The listing builds one solid part. Answer for the finished solid, in the listing's coordinates (mm). Coordinates: 2 decimals unless noted, no trailing zeros. Loops run counter-clockwise (first coordinate to the right, second up) from the corner with the lowest first, then second, coordinate; pieces in that order, holes last. Notation, with made-up numbers: M 53,60 L 92,60 A19 cw 92,77 Z; hole C 4,-20 d4. An arc over 180 degrees is marked long. Answer as a JSON object with one key per item and string values. Group by question number.
1. A cutting plane is placed at B-B on x = -4.5. State how many separate pieces and enclosed holes the cut face has, and give its area (3 significant figures).
2. Straight lines are drawn through the part: L1, parallel to X at y = 1.25, z = 16.5; L2, parallel to X at y = 1.3, z = 67; L3, parallel to X at y = 1.1, z = 97.5. For each, find the intervals that lie inside material, in ascending order.
3. Determine the mould class of faces 1 (the face through (25.75, 1.01, -105.07)), 2 (the face through (0, 2, -1)), 3 (the face through (-21.016, 0.986, 29.215)) for opening direction Z: released by +Z, released by -Z, zero draft, split by the parting line, or undercut.
4. A cutting plane is placed at A-A on z = 54. Give the vertices of the cut face in (x, y).
from build123d import *

# Parameters (mm, degrees)
SKETCH1_W            = 54.5
SKETCH1_H            = 213
BOSS_EXTRUDE1_DEPTH  = 2
M3_CLEARANCE_HOLE1_D = 3.6
CUT_EXTRUDE1_DEPTH   = 110.949135968
FILLET1_R            = 5


with BuildPart() as part:
    # Sketch1 → Boss-Extrude1 (new body)
    with BuildSketch(Plane(origin=(0, 0, 0), x_dir=(1, 0, 0), z_dir=(0, 1, 0))):
        Rectangle(SKETCH1_W, SKETCH1_H)
    extrude(amount=BOSS_EXTRUDE1_DEPTH)

    # M3 Clearance Hole1 (through all)
    with Locations(Plane(origin=(0, 2, 0), x_dir=(1, 0, 0), z_dir=(0, 1, 0))):
        with Locations((-21.25, 67), (-21.25, 31), (21.25, 67), (21.25, 31), (21.25, -31), (21.25, -67), (-21.25, -67), (-21.25, -31)):
            Hole(M3_CLEARANCE_HOLE1_D / 2)

    # Sketch5 → Cut-Extrude1 (cut, through all)
    with BuildSketch(Plane(origin=(0, 2, 0), x_dir=(1, 0, 0), z_dir=(0, 1, 0))):
        with BuildLine():
            Line((-18.25, 97.5), (-18.25, 80.5))
            ThreePointArc((-18.25, 80.5), (-20.25, 78.5), (-22.25, 80.5))
            Line((-22.25, 80.5), (-22.25, 97.5))
            ThreePointArc((-22.25, 97.5), (-20.25, 99.5), (-18.25, 97.5))
        make_face()
        with BuildLine():
            Line((18.25, 97.5), (18.25, 80.5))
            ThreePointArc((18.25, 80.5), (20.25, 78.5), (22.25, 80.5))
            Line((22.25, 80.5), (22.25, 97.5))
            ThreePointArc((22.25, 97.5), (20.25, 99.5), (18.25, 97.5))
        make_face()
        with BuildLine():
            Line((-10, 99.885191349), (10, 99.885191349))
            ThreePointArc((10, 99.885191349), (12, 97.885191349), (10, 95.885191349))
            Line((10, 95.885191349), (-10, 95.885191349))
            ThreePointArc((-10, 95.885191349), (-12, 97.885191349), (-10, 99.885191349))
        make_face()
        with BuildLine():
            Line((-10, 86.885191349), (10, 86.885191349))
            ThreePointArc((10, 86.885191349), (12, 84.885191349), (10, 82.885191349))
            Line((10, 82.885191349), (-10, 82.885191349))
            ThreePointArc((-10, 82.885191349), (-12, 84.885191349), (-10, 86.885191349))
        make_face()
        with BuildLine():
            Line((-10, 73.885191349), (10, 73.885191349))
            ThreePointArc((10, 73.885191349), (12, 71.885191349), (10, 69.885191349))
            Line((10, 69.885191349), (-10, 69.885191349))
            ThreePointArc((-10, 69.885191349), (-12, 71.885191349), (-10, 73.885191349))
        make_face()
        with BuildLine():
            Line((-10, 60.885191349), (10, 60.885191349))
            ThreePointArc((10, 60.885191349), (12, 58.885191349), (10, 56.885191349))
            Line((10, 56.885191349), (-10, 56.885191349))
            ThreePointArc((-10, 56.885191349), (-12, 58.885191349), (-10, 60.885191349))
        make_face()
        with BuildLine():
            Line((-10, 47.885191349), (10, 47.885191349))
            ThreePointArc((10, 47.885191349), (12, 45.885191349), (10, 43.885191349))
            Line((10, 43.885191349), (-10, 43.885191349))
            ThreePointArc((-10, 43.885191349), (-12, 45.885191349), (-10, 47.885191349))
        make_face()
        with BuildLine():
            Line((-10, 34.885191349), (10, 34.885191349))
            ThreePointArc((10, 34.885191349), (12, 32.885191349), (10, 30.885191349))
            Line((10, 30.885191349), (-10, 30.885191349))
            ThreePointArc((-10, 30.885191349), (-12, 32.885191349), (-10, 34.885191349))
        make_face()
        with BuildLine():
            Line((-10, 21.885191349), (10, 21.885191349))
            ThreePointArc((10, 21.885191349), (12, 19.885191349), (10, 17.885191349))
            Line((10, 17.885191349), (-10, 17.885191349))
            ThreePointArc((-10, 17.885191349), (-12, 19.885191349), (-10, 21.885191349))
        make_face()
        with BuildLine():
            Line((-10, 8.885191349), (10, 8.885191349))
            ThreePointArc((10, 8.885191349), (12, 6.885191349), (10, 4.885191349))
            Line((10, 4.885191349), (-10, 4.885191349))
            ThreePointArc((-10, 4.885191349), (-12, 6.885191349), (-10, 8.885191349))
        make_face()
        with BuildLine():
            Line((-19.25, 57.932734115), (-19.25, 40.067265885))
            ThreePointArc((-19.25, 40.067265885), (-21.25, 38.067265885), (-23.25, 40.067265885))
            Line((-23.25, 40.067265885), (-23.25, 57.932734115))
            ThreePointArc((-23.25, 57.932734115), (-21.25, 59.932734115), (-19.25, 57.932734115))
        make_face()
        with BuildLine():
            Line((-19.25, 22.533690779), (-19.25, 8.466309221))
            ThreePointArc((-19.25, 8.466309221), (-21.25, 6.466309221), (-23.25, 8.466309221))
            Line((-23.25, 8.466309221), (-23.25, 22.533690779))
            ThreePointArc((-23.25, 22.533690779), (-21.25, 24.533690779), (-19.25, 22.533690779))
        make_face()
        with BuildLine():
            Line((19.25, 57.932734115), (19.25, 40.067265885))
            ThreePointArc((19.25, 40.067265885), (21.25, 38.067265885), (23.25, 40.067265885))
            Line((23.25, 40.067265885), (23.25, 57.932734115))
            ThreePointArc((23.25, 57.932734115), (21.25, 59.932734115), (19.25, 57.932734115))
        make_face()
        with BuildLine():
            Line((19.25, 22.533690779), (19.25, 8.466309221))
            ThreePointArc((19.25, 8.466309221), (21.25, 6.466309221), (23.25, 8.466309221))
            Line((23.25, 8.466309221), (23.25, 22.533690779))
            ThreePointArc((23.25, 22.533690779), (21.25, 24.533690779), (19.25, 22.533690779))
        make_face()
        with BuildLine():
            Line((-18.25, -97.5), (-18.25, -80.5))
            ThreePointArc((-18.25, -80.5), (-20.25, -78.5), (-22.25, -80.5))
            Line((-22.25, -80.5), (-22.25, -97.5))
            ThreePointArc((-22.25, -97.5), (-20.25, -99.5), (-18.25, -97.5))
        make_face()
        with BuildLine():
            Line((18.25, -97.5), (18.25, -80.5))
            ThreePointArc((18.25, -80.5), (20.25, -78.5), (22.25, -80.5))
            Line((22.25, -80.5), (22.25, -97.5))
            ThreePointArc((22.25, -97.5), (20.25, -99.5), (18.25, -97.5))
        make_face()
        with BuildLine():
            Line((-10, -99.885191349), (10, -99.885191349))
            ThreePointArc((10, -99.885191349), (12, -97.885191349), (10, -95.885191349))
            Line((10, -95.885191349), (-10, -95.885191349))
            ThreePointArc((-10, -95.885191349), (-12, -97.885191349), (-10, -99.885191349))
        make_face()
        with BuildLine():
            Line((-10, -86.885191349), (10, -86.885191349))
            ThreePointArc((10, -86.885191349), (12, -84.885191349), (10, -82.885191349))
            Line((10, -82.885191349), (-10, -82.885191349))
            ThreePointArc((-10, -82.885191349), (-12, -84.885191349), (-10, -86.885191349))
        make_face()
        with BuildLine():
            Line((-10, -73.885191349), (10, -73.885191349))
            ThreePointArc((10, -73.885191349), (12, -71.885191349), (10, -69.885191349))
            Line((10, -69.885191349), (-10, -69.885191349))
            ThreePointArc((-10, -69.885191349), (-12, -71.885191349), (-10, -73.885191349))
        make_face()
        with BuildLine():
            Line((-10, -60.885191349), (10, -60.885191349))
            ThreePointArc((10, -60.885191349), (12, -58.885191349), (10, -56.885191349))
            Line((10, -56.885191349), (-10, -56.885191349))
            ThreePointArc((-10, -56.885191349), (-12, -58.885191349), (-10, -60.885191349))
        make_face()
        with BuildLine():
            Line((-10, -47.885191349), (10, -47.885191349))
            ThreePointArc((10, -47.885191349), (12, -45.885191349), (10, -43.885191349))
            Line((10, -43.885191349), (-10, -43.885191349))
            ThreePointArc((-10, -43.885191349), (-12, -45.885191349), (-10, -47.885191349))
        make_face()
        with BuildLine():
            Line((-10, -34.885191349), (10, -34.885191349))
            ThreePointArc((10, -34.885191349), (12, -32.885191349), (10, -30.885191349))
            Line((10, -30.885191349), (-10, -30.885191349))
            ThreePointArc((-10, -30.885191349), (-12, -32.885191349), (-10, -34.885191349))
        make_face()
        with BuildLine():
            Line((-10, -21.885191349), (10, -21.885191349))
            ThreePointArc((10, -21.885191349), (12, -19.885191349), (10, -17.885191349))
            Line((10, -17.885191349), (-10, -17.885191349))
            ThreePointArc((-10, -17.885191349), (-12, -19.885191349), (-10, -21.885191349))
        make_face()
        with BuildLine():
            Line((-10, -8.885191349), (10, -8.885191349))
            ThreePointArc((10, -8.885191349), (12, -6.885191349), (10, -4.885191349))
            Line((10, -4.885191349), (-10, -4.885191349))
            ThreePointArc((-10, -4.885191349), (-12, -6.885191349), (-10, -8.885191349))
        make_face()
        with BuildLine():
            Line((-19.25, -57.932734115), (-19.25, -40.067265885))
            ThreePointArc((-19.25, -40.067265885), (-21.25, -38.067265885), (-23.25, -40.067265885))
            Line((-23.25, -40.067265885), (-23.25, -57.932734115))
            ThreePointArc((-23.25, -57.932734115), (-21.25, -59.932734115), (-19.25, -57.932734115))
        make_face()
        with BuildLine():
            Line((-19.25, -22.533690779), (-19.25, -8.466309221))
            ThreePointArc((-19.25, -8.466309221), (-21.25, -6.466309221), (-23.25, -8.466309221))
            Line((-23.25, -8.466309221), (-23.25, -22.533690779))
            ThreePointArc((-23.25, -22.533690779), (-21.25, -24.533690779), (-19.25, -22.533690779))
        make_face()
        with BuildLine():
            Line((19.25, -57.932734115), (19.25, -40.067265885))
            ThreePointArc((19.25, -40.067265885), (21.25, -38.067265885), (23.25, -40.067265885))
            Line((23.25, -40.067265885), (23.25, -57.932734115))
            ThreePointArc((23.25, -57.932734115), (21.25, -59.932734115), (19.25, -57.932734115))
        make_face()
        with BuildLine():
            Line((19.25, -22.533690779), (19.25, -8.466309221))
            ThreePointArc((19.25, -8.466309221), (21.25, -6.466309221), (23.25, -8.466309221))
            Line((23.25, -8.466309221), (23.25, -22.533690779))
            ThreePointArc((23.25, -22.533690779), (21.25, -24.533690779), (19.25, -22.533690779))
        make_face()
    extrude(amount=-CUT_EXTRUDE1_DEPTH, mode=Mode.SUBTRACT)

    # Fillet1
    fillet1_edges = [part.edges().sort_by_distance(p)[0] for p in [
        (27.25, 1, 106.5),
        (-27.25, 1, 106.5),
        (-27.25, 1, -106.5),
        (27.25, 1, -106.5),
    ]]
    fillet(fillet1_edges, radius=FILLET1_R)


solid = part.part
From the geometry:
{
 "1": {"separate pieces": "17", "enclosed holes": "0", "area": "298 mm²"},
 "2": {"L1": "x = -27.25 to -23.25, -19.25 to 19.25, 23.25 to 27.25", "L2": "x = -27.25 to -23.05, -19.45 to 19.45, 23.05 to 27.25", "L3": "x = -27.25 to -22.25, -18.25 to -11.96, 11.96 to 18.25, 22.25 to 27.25"},
 "3": {"face 1": "released by -Z", "face 2": "zero draft", "face 3": "undercut"},
 "4": {"outline": "M -27.25,0 L -23.25,0 L -23.25,2 L -27.25,2 Z; M -19.25,0 L 19.25,0 L 19.25,2 L -19.25,2 Z; M 23.25,0 L 27.25,0 L 27.25,2 L 23.25,2 Z"}
}
